Could you check a few things on this model? Use its own coordinates, in mm. Give positions to 0.01 mm unless a question says otherwise; leave off trailing zeros. Loops run counter-clockwise (first coordinate to the right, second up) from the corner with the lowest first, then second, coordinate; pieces in that order, holes last. Notation, with made-up numbers: M 19,-5 L 27,-5 A19 ccw 27,19 Z; hole C -37.75,81 d6. An arc over 180 degrees is marked long. Return JSON: item names as keys, results as strings. Group by question number.
1. If we section it at C-C (y = 0.7): Write out the boundary of the cut face in (x, z).
2. Please list where these lines run through material, in increasing order: line 1 (Z direction, x = 0.5, y = 0.8); line 2 (Z direction, x = -2.75, y = 0.95); line 3 (X direction, y = 0.55, z = 0).
3. If we section it at B-B (x = 9.75): Write out the boundary of the cut face in (y, z), plus the area to 3 significant figures.
4. If we section it at D-D (z = -6): Write out the boundary of the cut face in (x, y).
5. If we mould it in two halves opening along Z, with no side actions, what happens to faces 1 (the flat face through (-6.566, 0.986, -8.798)), 2 (the cylindrical face through (0.9, 1.01, 2.86)), 3 (the cylindrical face through (0.795, 0.986, 25.846))? For each: +Z half, -Z half, draft (parallel to the pull), parting line (faces both ways), or undercut.
6. If we section it at A-A (z = 18): Write out the boundary of the cut face in (x, y), plus the area to 3 significant figures.
7. For pin 1 (1 mm diameter, centred on y = 1.5, z = 1, fed in from -X); pin 2 (4 mm diameter, centred on x = 0, z = -10, fed in from -Y), each with a flat end and sliding along its axis, tell me the tip position at first contact or that it passes through.
```python
from build123d import *

# Parameters (mm, degrees)
SKETCH_1_R          = 7.5
EXTRUDE_1_DEPTH     = 2
EXTRUDE_START       = -2
SKETCH_2_R          = 3
EXTRUDE_2_DEPTH     = 2
SKETCH_3_R          = 3
CUT_EXTRUDE_1_DEPTH = 2


with BuildPart() as part:
    # 草图1 → 凸台-拉伸1 (new body)
    # profile 1 of 2: a face of its own
    with BuildSketch(Plane(origin=(0, 0, 0), x_dir=(1, 0, 0), z_dir=(0, 1, 0))):
        Circle(SKETCH_1_R)
    # profile 2 of 2: a face of its own
    with BuildSketch(Plane(origin=(0, 0, 0), x_dir=(1, 0, 0), z_dir=(0, 1, 0))):
        with BuildLine():
            ThreePointArc((17.5, 0), (10.160196291, 14.248523128), (-5.702332724, 16.544890495))
            Line((-5.702332724, 16.544890495), (-7.453841227, 0.830813432))
            ThreePointArc((-7.453841227, 0.830813432), (-5.000944874, 5.589324679), (0, 7.5))
            ThreePointArc((0, 7.5), (3.750000007, 6.495190524), (6.495190536, 3.749999986))
            ThreePointArc((6.495190536, 3.749999986), (7.244443699, 1.94114283), (7.5, 0))
            ThreePointArc((7.5, 0), (7.244443692, -1.941142857), (6.495190509, -3.750000034))
            ThreePointArc((6.495190509, -3.750000034), (2.340024706, -7.125607649), (-3.007415076, -6.870622574))
            Line((-3.007415076, -6.870622574), (11.47712911, -13.210810248))
            ThreePointArc((11.47712911, -13.210810248), (15.923249659, -7.25948485), (17.5, 0))
        make_face()
        with BuildLine():
            ThreePointArc((11.160254038, -5), (8.013206444, -7.414814571), (6.495190509, -3.750000034))
            ThreePointArc((6.495190509, -3.750000034), (9.307301631, -2.585185429), (11.160254038, -5))
        make_face(mode=Mode.SUBTRACT)
        with BuildLine():
            ThreePointArc((11.160254038, 5), (9.307301658, 2.585185436), (6.495190536, 3.749999986))
            ThreePointArc((6.495190536, 3.749999986), (8.013206417, 7.414814564), (11.160254038, 5))
        make_face(mode=Mode.SUBTRACT)
        with BuildLine():
            ThreePointArc((2.5, 10), (1.767766953, 8.232233047), (0, 7.5))
            ThreePointArc((0, 7.5), (-1.767766953, 11.767766953), (2.5, 10))
        make_face(mode=Mode.SUBTRACT)
    extrude(amount=EXTRUDE_1_DEPTH)

    # 草图2 → 凸台-拉伸2 (add)
    with BuildSketch(Plane(origin=(0, 2, 0), x_dir=(1, 0, 0), z_dir=(0, 1, 0)).offset(EXTRUDE_START)):
        with BuildLine():
            ThreePointArc((-3.007415076, -6.870622574), (-6.018851538, -4.474754313), (-7.445705299, -0.90081774))
            Line((-7.445705299, -0.90081774), (-5.164424019, -19.756738712))
            ThreePointArc((-5.164424019, -19.756738712), (0.924105936, -25.862847589), (8.318844201, -21.427466138))
            Line((8.318844201, -21.427466138), (11.47712911, -13.210810248))
            Line((11.47712911, -13.210810248), (-3.007415076, -6.870622574))
        make_face()
        with Locations(Location((1.784900926, -18.915975489, 0), (0, 0, 270))):
            Circle(SKETCH_2_R, mode=Mode.SUBTRACT)
    extrude(amount=EXTRUDE_2_DEPTH)

    # 草图3 → 切除-拉伸1 (cut)
    with BuildSketch(Plane(origin=(0, 2, 0), x_dir=(1, 0, 0), z_dir=(0, 1, 0))):
        with Locations(Location((0, 0, 0), (0, 0, 270))):
            Circle(SKETCH_3_R)
    extrude(amount=-CUT_EXTRUDE_1_DEPTH, mode=Mode.SUBTRACT)


solid = part.part
```
Answer:
{
 "1": {"outline": "M -7.45,-0.83 L -5.7,-16.54 A17.5 ccw 11.48,13.21 L 8.32,21.43 A7 ccw -5.16,19.76 L -7.45,0.9 A7.5 ccw Z; hole C 0,0 d6; hole C 0,-10 d5; hole C 1.78,18.92 d6; hole C 8.66,-5 d5; hole C 8.66,5 d5"},
 "2": {"line 1": "z = -17.49 to -12.45, -7.55 to -2.96, 2.96 to 16.21, 21.63 to 25.8", "line 2": "z = -17.28 to -1.2, 1.2 to 24.25", "line 3": "x = -7.5 to -3, 3 to 17.5"},
 "3": {"outline": "M 0,-14.53 L 2,-14.53 L 2,-7.25 L 0,-7.25 Z; M 0,-2.75 L 2,-2.75 L 2,2.75 L 0,2.75 Z; M 0,7.25 L 2,7.25 L 2,17.7 L 0,17.7 Z", "area": "46.5 mm²"},
 "4": {"outline": "M -6.88,0 L 6.37,0 L 6.37,2 L -6.88,2 Z; M 10.95,0 L 16.44,0 L 16.44,2 L 10.95,2 Z"},
 "5": {"face 1": "-Z half", "face 2": "undercut", "face 3": "+Z half"},
 "6": {"outline": "M -5.38,0 L -1.07,0 L -1.07,2 L -5.38,2 Z; M 4.64,0 L 9.64,0 L 9.64,2 L 4.64,2 Z", "area": "18.6 mm²"},
 "7": {"pin 1": "stops at x = -7.48", "pin 2": "passes through"}
}
